from build123d import *

# Parameters (mm, degrees)
F0_R     = 2.5
F0_R_2   = 11
F1_DEPTH = 4
F0_R_3   = 7
F0_R_4   = 4
F2_DEPTH = 13
F3_DEPTH = 10
F4_R     = 1
F5_DEPTH = 8
F6_SIZE  = 0.2
F7_SIZE  = 0.2
F8_SIZE  = 0.2


with BuildPart() as f1:
    # F0 (on Front) → F1 (new body)
    with BuildSketch(Plane.XZ):
        with BuildLine():
            Line((-20.369007, -3.539129), (-6.934932, -11.582604))
            ThreePointArc((-6.934932, -11.582604), (0, -13.5), (6.934932, -11.582604))
            Line((6.934932, -11.582604), (20.369007, -3.539129))
            ThreePointArc((20.369007, -3.539129), (22.375, 0), (20.369007, 3.539129))
            Line((20.369007, 3.539129), (6.934932, 11.582604))
            ThreePointArc((6.934932, 11.582604), (0, 13.5), (-6.934932, 11.582604))
            Line((-6.934932, 11.582604), (-20.369007, 3.539129))
            ThreePointArc((-20.369007, 3.539129), (-22.375, 0), (-20.369007, -3.539129))
        make_face()
        with Locations((-18.25, 0)):
            Circle(F0_R, mode=Mode.SUBTRACT)
        Circle(F0_R_2, mode=Mode.SUBTRACT)
        with Locations((18.25, 0)):
            Circle(F0_R, mode=Mode.SUBTRACT)
    extrude(amount=F1_DEPTH)



with BuildPart() as f2:
    # F0 (on Front) → F2 (new body)
    with BuildSketch(Plane.XZ):
        Circle(F0_R_3)
        Circle(F0_R_4, mode=Mode.SUBTRACT)
    extrude(amount=F2_DEPTH)


with BuildPart() as f1_1:
    add(f1.part)

    add(f2.part)  # F3 merges F2
    # F0 (on Front) → F3 (join)
    with BuildSketch(Plane.XZ):
        Circle(F0_R_2)
        Circle(F0_R_3, mode=Mode.SUBTRACT)
    extrude(amount=F3_DEPTH)

    # F4 (on Right) → F5 (cut)
    with BuildSketch(Plane.YZ):
        with Locations((-11.5, 0)):
            Circle(F4_R)
    extrude(amount=F5_DEPTH, mode=Mode.SUBTRACT)

    # F6
    f6_edges = [f1_1.edges().sort_by_distance(p)[0] for p in [
        (-11, -10, 0),
    ]]
    chamfer(f6_edges, length=F6_SIZE)

    # F7
    f7_edges = [f1_1.edges().sort_by_distance(p)[0] for p in [
        (-7, -13, 0),
    ]]
    chamfer(f7_edges, length=F7_SIZE)

    # F8
    f8_edges = [f1_1.edges().sort_by_distance(p)[0] for p in [
        (13.651969, -4, -7.560867),
        (13.651969, -4, 7.560867),
        (22.375, -4, 0),
        (0, -4, -13.5),
        (0, -4, 13.5),
        (-13.651969, -4, 7.560867),
        (-13.651969, -4, -7.560867),
        (-22.375, -4, 0),
    ]]
    chamfer(f8_edges, length=F8_SIZE)


solid = f1_1.part
Verification items for the finished model (mm, model axes). A direction names the side the tool comes from. Give positions to 0.01 mm unless a question says otherwise; leave off trailing zeros. Loops run counter-clockwise (first coordinate to the right, second up) from the corner with the lowest first, then second, coordinate; pieces in that order, holes last.
1) Thickness scan on line 1 along Z through (x, y) = (0, -7.25); line 2 along Y through (x, z) = (-9.5, 3.5); line 3 along Z through (x, y) = (-18.25, -1.8). Record the ranges inside material, lowest first.
2) Set-up check for faces 1 (the cylindrical face through (-2.38, -6.86, -10.74)), 2 (the cylindrical face through (22.375, -1.873, -0.06)): record each of +Z, -Z, +X, -X, +Y, -Y from which the full face is reachable in a straight line by a thin tool's end or side.
3) Depth check by flat-ended pin: pin 1 Ø4 at (x, y) = (-9, -11) entering from -Z; pin 2 Ø1 at (x, y) = (10.5, -7.5) entering from -Z; pin 3 Ø4 at (x, z) = (11, -4.5) entering from -Y. Enter the tip coordinate at first touch or a pass-through.
4) Sectioned sample at C-C, the plane y = -1.25. Enter the section's corners in (x, z) (3 decimals).
5) Draft check along X on faces 3 (the cylindrical face through (15.752, -1.972, 0.11)), 4 (the cylindrical face through (-0.1, -1.9, -13.5)), 5 (the flat face through (3, -13, -3)). Enter one of: pulls with the +X half, pulls with the -X half, needs draft (parallel to the pull), parting line crosses it, or undercut.
6) Sectioned sample at D-D, the plane y = -8. Enter the section's corners in (x, z).
7) Sectioned sample at B-B, the plane x = 0. Enter the section's corners in (y, z), then the cut area to 3 significant figures.
8) Sectioned sample at A-A, the plane z = 0. Count the separate pieces of the cut face and the enclosed holes in it, then the cut area to 3 significant figures.
Answers:
1. line 1: z = -11 to -4, 4 to 11
1. line 2: y = -10 to 0
1. line 3: z = -4.81 to -2.5, 2.5 to 4.81
2. face 1: -Y
2. face 2: +X, +Y, -Y
3. pin 1: stops at z = -8.14
3. pin 2: stops at z = -4.58
3. pin 3: stops at y = -10
4. outline: (-20.369, -3.539) - (-6.935, -11.583) arc R13.5 ccw to (6.935, -11.583) - (20.369, -3.539) arc R4.125 ccw to (20.369, 3.539) - (6.935, 11.583) arc R13.5 ccw to (-6.935, 11.583) - (-20.369, 3.539) arc R4.125 ccw to start; hole circle Ø5 at (-18.25, 0); hole circle Ø8 at (0, 0); hole circle Ø5 at (18.25, 0)
5. face 3: undercut
5. face 4: parting line crosses it
5. face 5: needs draft
6. outline: circle Ø22 at (0, 0); hole circle Ø8 at (0, 0)
7. outline: (-13, -6.8) - (-12.8, -7) - (-10, -7) - (-10, -10.8) - (-9.8, -11) - (-4, -11) - (-4, -13.3) - (-3.8, -13.5) - (0, -13.5) - (0, -4) - (-13, -4) - close; (-13, 4) - (0, 4) - (0, 13.5) - (-3.8, 13.5) - (-4, 13.3) - (-4, 11) - (-9.8, 11) - (-10, 10.8) - (-10, 7) - (-12.8, 7) - (-13, 6.8) - close
7. area: 178 mm2
8. separate pieces: 5
8. enclosed holes: 0
8. area: 203 mm2
